Input: part model. Units: mm. Frame: model coordinates. Face numbers are marked on the shaded views. Coordinates: 2 decimals unless noted, no trailing zeros. Write each loop counter-clockwise with the first axis right and the second up, starting at its lowest first coordinate (ties: lowest second). Pieces come first, ordered by that corner, then holes. Notation, with made-up numbers: (-39.75, -3) - (-23.75, -3) arc R18 cw to (-23.75, 2) - close; hole circle Ø6 at (21.5, 22). An arc over 180 degrees is marked (long way). Use CSV: the item, a comma, the result in double quotes.
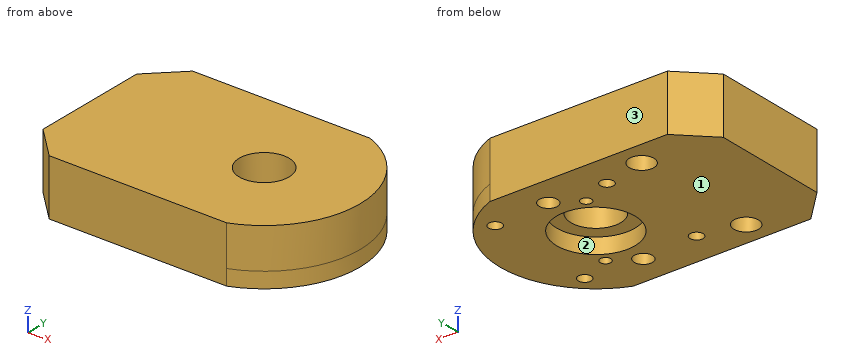
```python
from build123d import *

# Parameters (mm, degrees)
ESQUISSE1_R             = 1.98
ESQUISSE1_R_2           = 6.3
ESQUISSE1_R_3           = 1.475
ESQUISSE1_R_4           = 1.05
ESQUISSE1_R_5           = 0.85
BOSS_EXTRU_2_DEPTH      = 2.5
BOSS_EXTRU_3_DEPTH      = 6.5
ESQUISSE3_R             = 4
ENL_V_MAT_EXTRU_1_DEPTH = 10


with BuildPart() as part:
    # Esquisse1 → Boss.-Extru.2 (new body)
    with BuildSketch(Plane.XY):
        with BuildLine():
            Line((22.5, 28.77), (5, 28.77))
            Line((5, 28.77), (0, 23.77))
            Line((0, 23.77), (0, 5))
            Line((0, 5), (5, 0))
            Line((5, 0), (22.5, 0))
            Line((22.5, 0), (33.5, 0))
            ThreePointArc((33.5, 0), (43.400591709, 14.385), (33.5, 28.77))
            Line((33.5, 28.77), (22.5, 28.77))
        make_face()
        with Locations((12.25, 3.905)):
            Circle(ESQUISSE1_R, mode=Mode.SUBTRACT)
        with Locations((12.25, 24.865)):
            Circle(ESQUISSE1_R, mode=Mode.SUBTRACT)
        with Locations((28, 14.385)):
            Circle(ESQUISSE1_R_2, mode=Mode.SUBTRACT)
        with Locations((28, 4.86)):
            Circle(ESQUISSE1_R_3, mode=Mode.SUBTRACT)
        with Locations((28, 23.91)):
            Circle(ESQUISSE1_R_3, mode=Mode.SUBTRACT)
        with Locations((36.980256121, 5.404743879)):
            Circle(ESQUISSE1_R_4, mode=Mode.SUBTRACT)
        with Locations((36.980256121, 23.365256121)):
            Circle(ESQUISSE1_R_4, mode=Mode.SUBTRACT)
        with Locations((19.019743879, 23.365256121)):
            Circle(ESQUISSE1_R_4, mode=Mode.SUBTRACT)
        with Locations((19.019743879, 5.404743879)):
            Circle(ESQUISSE1_R_4, mode=Mode.SUBTRACT)
        with Locations((24, 21.31320323)):
            Circle(ESQUISSE1_R_5, mode=Mode.SUBTRACT)
        with Locations((32, 7.45679677)):
            Circle(ESQUISSE1_R_5, mode=Mode.SUBTRACT)
    extrude(amount=BOSS_EXTRU_2_DEPTH)

    # Esquisse2 → Boss.-Extru.3 (add)
    with BuildSketch(Plane.XY.offset(2.5)):
        with BuildLine():
            Line((5, 28.77), (33.5, 28.77))
            ThreePointArc((33.5, 28.77), (43.400493129, 14.385), (33.5, 0))
            Line((33.5, 0), (5, 0))
            Line((5, 0), (0, 5))
            Line((0, 5), (0, 23.77))
            Line((0, 23.77), (5, 28.77))
        make_face()
    extrude(amount=BOSS_EXTRU_3_DEPTH)

    # Esquisse3 → Enlèv. mat.-Extru.1 (cut)
    with BuildSketch(Plane.XY.offset(9)):
        with Locations((27.999846655, 14.385)):
            Circle(ESQUISSE3_R)
    extrude(amount=-ENL_V_MAT_EXTRU_1_DEPTH, mode=Mode.SUBTRACT)


solid = part.part
```
(1) Ray query, probe 1 along Y at (x, z) = (12.25, 1.25) (3 decimals); probe 2 along Y at (x, z) = (37, 1); probe 3 along X at (y, z) = (14.25, 2.25). Return the intervals inside material, ascending. Write a range as from..to.
Check values:
probe 1,"0..1.925, 5.885..22.885, 26.845..28.77"
probe 2,"1.89..4.35, 6.45..22.32, 24.42..26.88"
probe 3,"0..21.7, 34.3..43.4"
(2) Cut plane D-D on z = 6. Return loops of the section in (x, y) (3 decimals), and give its area (3 significant figures).
Check values:
outline,"(0, 5) - (5, 0) - (33.5, 0) arc R15.401 ccw to (33.5, 28.77) - (5, 28.77) - (0, 23.77) - close; hole circle Ø8 at (28, 14.385)"
area,"1,100 mm^2"
(3) Draft query along Y for the marked faces 1, 2 and 3. Return one class per face: pulls with the +Y half, pulls with the -Y half, needs draft (parallel to the pull), parting line crosses it, or undercut.
Check values:
face 1,"needs draft"
face 2,"undercut"
face 3,"pulls with the +Y half"
(4) Cut plane A-A on x = 28. Return loops of the section in (y, z) (3 decimals).
Check values:
outline,"(0, 0) - (3.385, 0) - (3.385, 2.5) - (6.335, 2.5) - (6.335, 0) - (8.085, 0) - (8.085, 2.5) - (10.385, 2.5) - (10.385, 9) - (0, 9) - close; (18.385, 2.5) - (20.685, 2.5) - (20.685, 0) - (22.435, 0) - (22.435, 2.5) - (25.385, 2.5) - (25.385, 0) - (28.77, 0) - (28.77, 9) - (18.385, 9) - close"
(5) Cut plane B-B on x = 12.25. Return loops of the section in (y, z) (3 decimals).
Check values:
outline,"(0, 0) - (1.925, 0) - (1.925, 2.5) - (5.885, 2.5) - (5.885, 0) - (22.885, 0) - (22.885, 2.5) - (26.845, 2.5) - (26.845, 0) - (28.77, 0) - (28.77, 9) - (0, 9) - close"
(6) Pin query (flat end, axial travel): pin 1 Ø1.1 at (x, y) = (19, 23) entering from -Z; pin 2 Ø2 at (y, z) = (16.5, 2) entering from +X. Return the tip coordinate at first contact, or that it passes through.
Check values:
pin 1,"z = 2.5"
pin 2,"x = 43.36"
